Read the model definition and answer for the solid it produces. Units are mm, in the model's axes. Face numbers are marked on the shaded views. A direction names the side the tool comes from. Give positions to 0.01 mm unless a question says otherwise; leave off trailing zeros. Loops run counter-clockwise (first coordinate to the right, second up) from the corner with the lowest first, then second, coordinate; pieces in that order, holes last. Notation, with made-up numbers: (73.5, 40.25) -> (87.5, 40.25) arc R24 cw to (87.5, 61.25) -> close; hole circle Ø10 at (27.25, -36). An arc over 180 degrees is marked (long way). Answer as CSV lines item,"result". Start each with the question number.
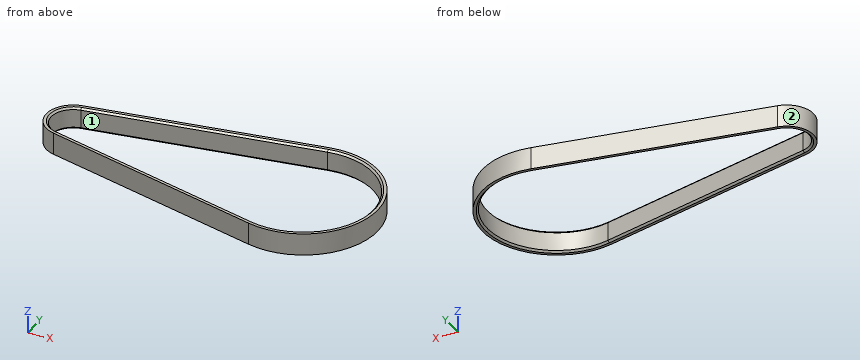
Autodesk Inventor part; units mm, degrees
ref_plane "YZ Plane" through (0, 0, 0) normal (1, 0, 0) x (0, 1, 0)
ref_plane "XZ Plane" through (0, 0, 0) normal (0, 1, 0) x (-1, 0, 0)
ref_plane "XY Plane" through (0, 0, 0) normal (0, 0, 1) x (1, 0, 0)
sketch "Sketch1" plane through (0, 0, 0) normal (0, 0, 1) x (1, 0, 0)
  arc A0 (-1.2105, 5.8766) -> (-1.2105, -5.8766) centre (0, 0) ccw
  arc A1 (59.8885, -18.4624) -> (59.8885, 18.4624) centre (63.6915, 0) ccw
  line L0 (-1.2105, 5.8766) -> (59.8885, 18.4624)
  line L1 (-1.2105, -5.8766) -> (59.8885, -18.4624)
  line L2 (59.6262, 19.7356) -> (-1.4728, 7.1499)
  arc A2 (-1.4728, 7.1499) -> (-1.4728, -7.1499) centre (0, 0) ccw
  line L3 (-1.4728, -7.1499) -> (59.6262, -19.7356)
  arc A3 (59.6262, -19.7356) -> (59.6262, 19.7356) centre (63.6915, 0) ccw
  dimension "d0" = 12
  dimension "d1" = 37.7
  dimension "d3" = 1.3
  dimension "d9" = 63.6915
extrude "Extrusion1" add sketch "Sketch1" along normal mid plane 6
chamfer "Chamfer1" distance 0.5 angle 45 8 edges at (-6, 0, 3) (29.339, 12.1695, 3) (82.5415, 0, 3) (29.339, -12.1695, 3) (-6, 0, -3) (29.339, -12.1695, -3) (82.5415, 0, -3) (29.339, 12.1695, -3)
properties part number "Tandriem16naar60T" material "Rubber"
(1) Find the intervals of material crossed by line 1 along Y through (x, z) = (30, 0.3); line 2 along Y through (x, z) = (43, -2.3); line 3 along X through (y, z) = (2.5, -2.7), in increasing order. Write a range as from..to.
(2) Each of these flat-tipped pins is pushed along its axis until it touches: P1, Ø1.5, axis at x = 37.5, z = 1.5, coming from the -Y side; P2, Ø2, axis at x = 14.5, z = 0.5, coming from the +Y side; P3, Ø2, axis at x = 6.5, z = 0.5, coming from the -Y side. Where does it stop, or does it pass through?
(3) Find section B-B on z = -0.25. Write down the section's boundary in (x, y), then the cut area to 3 significant figures.
(4) Find section A-A on y = 0. Write down the section's boundary in (x, z).
(5) A tool of negligible diameter and unlimited length cuts with its end or side. For the marked faces 1 and 2, from which of +Z, -Z, +X, -X, +Y, -Y can it reach the whole face along a straight path? Write none if from no direction.
(6) Find section C-C on x = 12.5. Write down the section's boundary in (y, z).
Answer block:
1,line 1,"y = -13.63..-12.31, 12.31..13.63"
1,line 2,"y = -16.31..-14.98, 14.98..16.31"
1,line 3,"x = -6.86..-5.67, 82.58..83.69"
2,P1,"stops at y = -15.33"
2,P2,"stops at y = 10.65"
2,P3,"stops at y = -9"
3,outline,"(-1.47, -7.15) -> (59.63, -19.74) arc R20.15 ccw (long way) to (59.63, 19.74) -> (-1.47, 7.15) arc R7.3 ccw to start; hole (-1.21, -5.88) -> (59.89, -18.46) arc R18.85 ccw (long way) to (59.89, 18.46) -> (-1.21, 5.88) arc R6 ccw to start"
3,area,"276 mm2"
4,outline,"(-7.3, -3) -> (-6.5, -3) -> (-6, -2.5) -> (-6, 2.5) -> (-6.5, 3) -> (-7.3, 3) -> close; (82.54, -2.5) -> (83.04, -3) -> (83.84, -3) -> (83.84, 3) -> (83.04, 3) -> (82.54, 2.5) -> close"
5,face 1,"+Z, -Z"
5,face 2,"+Z, -Z, -X"
6,outline,"(-10.03, -3) -> (-9.21, -3) -> (-8.7, -2.5) -> (-8.7, 2.5) -> (-9.21, 3) -> (-10.03, 3) -> close; (8.7, -2.5) -> (9.21, -3) -> (10.03, -3) -> (10.03, 3) -> (9.21, 3) -> (8.7, 2.5) -> close"
